from build123d import *

# Parameters (mm, degrees)
F0_W      = 117.348
F0_H      = 63.5
F1_DEPTH  = 50.8
F2_W      = 41.148
F2_H      = 19.304
F3_DEPTH  = 50.801
F4_W      = 56.896
F4_H      = 12.7
F5_DEPTH  = 50.801
F6_R      = 9.525
F7_DEPTH  = 50.801
F8_W      = 15.748
F8_H      = 12.7
F9_DEPTH  = 117.349
F10_W     = 35.052
F10_H     = 12.7
F11_DEPTH = 76.201
F12_W     = 15.748
F12_H     = 38.1
F13_DEPTH = 76.201
F14_W     = 15.748
F14_H     = 31.496
F15_DEPTH = 117.349


with BuildPart() as f1:
    # F0 (on Front) → F1 (new body)
    with BuildSketch(Plane.XZ):
        Rectangle(F0_W, F0_H)
    extrude(amount=F1_DEPTH)

    # F2 (on face) → F3 (cut, through all)
    with BuildSketch(Plane.XZ.offset(50.8)):
        with Locations((38.1, 22.098)):
            Rectangle(F2_W, F2_H)
    extrude(amount=-F3_DEPTH, mode=Mode.SUBTRACT)

    # F4 (on face) → F5 (cut, through all)
    with BuildSketch(Plane.XZ.offset(50.8)):
        with Locations((-30.226, -25.4)):
            Rectangle(F4_W, F4_H)
    extrude(amount=-F5_DEPTH, mode=Mode.SUBTRACT)

    # F6 (on face) → F7 (cut, through all)
    with BuildSketch(Plane.XZ.offset(50.8)):
        with Locations((-26.67, -0.254)):
            Circle(F6_R)
    extrude(amount=-F7_DEPTH, mode=Mode.SUBTRACT)

    # F8 (on face) → F9 (cut, through all)
    with BuildSketch(Plane.YZ.offset(58.674)):
        with Locations((-7.874, -25.4)):
            Rectangle(F8_W, F8_H)
    extrude(amount=-F9_DEPTH, mode=Mode.SUBTRACT)

    # F10 (on face) → F11 (cut, through all)
    with BuildSketch(Plane.YZ.offset(17.526)):
        with Locations((-33.274, 25.4)):
            Rectangle(F10_W, F10_H)
    extrude(amount=-F11_DEPTH, mode=Mode.SUBTRACT)

    # F12 (on face) → F13 (cut, through all)
    with BuildSketch(Plane.YZ.offset(17.526)):
        with Locations((-42.926, 0)):
            Rectangle(F12_W, F12_H)
    extrude(amount=-F13_DEPTH, mode=Mode.SUBTRACT)

    # F14 (on face) → F15 (cut, through all)
    with BuildSketch(Plane.YZ.offset(58.674)):
        with Locations((-42.926, -3.302)):
            Rectangle(F14_W, F14_H)
    extrude(amount=-F15_DEPTH, mode=Mode.SUBTRACT)


solid = f1.part
Can you work these out from the model? Positions are in its coordinate system, mm. A direction names the side the tool comes from. Give positions to 0.01 mm unless a question says otherwise; leave off trailing zeros. Loops run counter-clockwise (first coordinate to the right, second up) from the corner with the lowest first, then second, coordinate; pieces in that order, holes last. Notation, with made-up numbers: (9, 49.5) - (40, 49.5) arc R29 cw to (40, 71.5) - close; hole circle Ø11 at (-39.5, 15). An arc over 180 degrees is marked (long way). Return JSON: item names as keys, results as strings.
1. I want a section at C-C on x = -39.5. Please give me the cut outline in (y, z), and give its area (3 significant figures).
Output values:
{"outline": "(-35.05, -19.05) - (0, -19.05) - (0, 31.75) - (-15.75, 31.75) - (-15.75, 19.05) - (-35.05, 19.05) - close", "area": "1,540 mm²"}
2. If I drill on line 1 (Z direction, x = -26.67, y = -25); line 2 (Z direction, x = -26.67, y = -11); line 3 (Y direction, x = -32.5, z = -16), over which ranges is the centre line in solid material (lowest first)?
Output values:
{"line 1": "z = -19.05 to -9.78, 9.27 to 19.05", "line 2": "z = -19.05 to -9.78, 9.27 to 31.75", "line 3": "y = -35.05 to 0"}
3. I want a section at A-A on x = -26.67. Please give me the cut outline in (y, z).
Output values:
{"outline": "(-35.05, -19.05) - (0, -19.05) - (0, -9.78) - (-35.05, -9.78) - close; (-35.05, 9.27) - (0, 9.27) - (0, 31.75) - (-15.75, 31.75) - (-15.75, 19.05) - (-35.05, 19.05) - close"}
4. I want a section at D-D on y = -21. Please give me the cut outline in (x, z) (3 decimals).
Output values:
{"outline": "(-58.674, -19.05) - (-1.778, -19.05) - (-1.778, -31.75) - (58.674, -31.75) - (58.674, 12.446) - (17.526, 12.446) - (17.526, 19.05) - (-58.674, 19.05) - close; hole circle Ø19.05 at (-26.67, -0.254)"}
5. I want a section at B-B on z = -7. Please give me the cut outline in (x, y), and give its area (3 significant figures).
Output values:
{"outline": "(-58.67, -35.05) - (-33.39, -35.05) - (-33.39, 0) - (-58.67, 0) - close; (-19.95, -35.05) - (58.67, -35.05) - (58.67, 0) - (-19.95, 0) - close", "area": "3,640 mm²"}
6. We'd pull the mould along X, two halves only. Please class faces 4 (the face through (-58.674, -17, 6)), 5 (the face through (-20, -15.748, 25)), 6 (the face through (-33.69, -17.771, 6.183)): +X half, -X half, draft (parallel to the pull), parting line (faces both ways), or undercut.
Output values:
{"face 4": "-X half", "face 5": "draft", "face 6": "undercut"}
7. I'm going to push flat-ended pins straight in: pin 1 Ø1 at (x, y) = (36.5, -27.5) entering from +Z; pin 2 Ø11.5 at (x, z) = (-18.5, 9) entering from -Y; pin 3 Ø4 at (x, z) = (-14, 28.5) entering from -Y; pin 4 Ø5 at (y, z) = (-25, 22) entering from -X. Where does each tip first touch, or does it pass through?
Output values:
{"pin 1": "stops at z = 12.45", "pin 2": "stops at y = -35.05", "pin 3": "stops at y = -15.75", "pin 4": "passes through"}
8. For faces 1 (the face through (38, -18, 12.446)), 2 (the face through (-1.778, -34, -25)), 3 (the face through (1, -35.052, 0)), which set-ups out of +Z, -Z, +X, -X, +Y, -Y let a thin tool reach every point of the face, with its end or its side?
Output values:
{"face 1": "+Z, +X, +Y, -Y", "face 2": "-Z, -X, +Y, -Y", "face 3": "+Z, +X, -X, -Y"}
